from build123d import *

# Parameters (mm, degrees)
F1_DEPTH = 10
F2_DEPTH = 8
F3_DEPTH = 5


with BuildPart() as f1:
    # F0 (on Front) → F1 (new body, symmetric)
    with BuildSketch(Plane.XZ):
        with BuildLine():
            ThreePointArc((3.989783, 27.714286), (0, 24), (-3.989783, 27.714286))
            ThreePointArc((-3.989783, 27.714286), (-9.576564, 26.311393), (-14.758048, 23.794958))
            ThreePointArc((-14.758048, 23.794958), (-15.426903, 18.385067), (-20.87075, 18.665792))
            ThreePointArc((-20.87075, 18.665792), (-24.248711, 14), (-26.600425, 8.741704))
            ThreePointArc((-26.600425, 8.741704), (-23.635386, 4.167556), (-27.986062, 0.883366))
            ThreePointArc((-27.986062, 0.883366), (-27.574617, -4.862149), (-25.996167, -10.40189))
            ThreePointArc((-25.996167, -10.40189), (-20.78461, -12), (-22.006384, -17.312396))
            ThreePointArc((-22.006384, -17.312396), (-17.998053, -21.449244), (-13.228013, -24.678324))
            ThreePointArc((-13.228013, -24.678324), (-8.208483, -22.552623), (-5.729674, -27.407496))
            ThreePointArc((-5.729674, -27.407496), (0, -28), (5.729674, -27.407496))
            ThreePointArc((5.729674, -27.407496), (8.208483, -22.552623), (13.228013, -24.678324))
            ThreePointArc((13.228013, -24.678324), (17.998053, -21.449244), (22.006384, -17.312396))
            ThreePointArc((22.006384, -17.312396), (20.78461, -12), (25.996167, -10.40189))
            ThreePointArc((25.996167, -10.40189), (27.574617, -4.862149), (27.986062, 0.883366))
            ThreePointArc((27.986062, 0.883366), (23.635386, 4.167556), (26.600425, 8.741704))
            ThreePointArc((26.600425, 8.741704), (24.248711, 14), (20.87075, 18.665792))
            ThreePointArc((20.87075, 18.665792), (15.426903, 18.385067), (14.758048, 23.794958))
            ThreePointArc((14.758048, 23.794958), (9.576564, 26.311393), (3.989783, 27.714286))
        make_face()
        with BuildLine():
            ThreePointArc((2, 19.899749), (0, -20), (-2, 19.899749))
            Line((-2, 19.899749), (-2, 21.899749))
            Line((-2, 21.899749), (2, 21.899749))
            Line((2, 21.899749), (2, 19.899749))
        make_face(mode=Mode.SUBTRACT)
    extrude(amount=F1_DEPTH, both=True)



with BuildPart() as f2:
    # F0 (on Front) → F2 (new body, symmetric)
    with BuildSketch(Plane.XZ):
        with BuildLine():
            Line((-10.825318, 78.25), (-15.155445, 80.75))
            ThreePointArc((-15.155445, 80.75), (-17.338404, 74.372706), (-16.949042, 67.643398))
            ThreePointArc((-16.949042, 67.643398), (0, 54.5), (16.949042, 67.643398))
            ThreePointArc((16.949042, 67.643398), (17.338404, 74.372706), (15.155445, 80.75))
            Line((15.155445, 80.75), (10.825318, 78.25))
            ThreePointArc((10.825318, 78.25), (0, 59.5), (-10.825318, 78.25))
        make_face()
        with BuildLine():
            ThreePointArc((-50.10638, -48.5), (-47.198385, -27.25), (-67.055422, -19.143398))
            ThreePointArc((-67.055422, -19.143398), (-73.077855, -22.170855), (-77.509274, -27.25))
            Line((-77.509274, -27.25), (-73.179147, -29.75))
            ThreePointArc((-73.179147, -29.75), (-51.528512, -29.75), (-62.353829, -48.5))
            Line((-62.353829, -48.5), (-62.353829, -53.5))
            ThreePointArc((-62.353829, -53.5), (-55.739451, -52.201852), (-50.10638, -48.5))
        make_face()
        with BuildLine():
            ThreePointArc((77.509274, -27.25), (73.077855, -22.170855), (67.055422, -19.143398))
            ThreePointArc((67.055422, -19.143398), (47.198385, -27.25), (50.10638, -48.5))
            ThreePointArc((50.10638, -48.5), (55.739451, -52.201852), (62.353829, -53.5))
            Line((62.353829, -53.5), (62.353829, -48.5))
            ThreePointArc((62.353829, -48.5), (51.528512, -29.75), (73.179147, -29.75))
            Line((73.179147, -29.75), (77.509274, -27.25))
        make_face()
    extrude(amount=F2_DEPTH, both=True)


with BuildPart() as f1_1:
    add(f1.part)

    add(f2.part)  # F3 merges F2
    # F0 (on Front) → F3 (join, symmetric)
    with BuildSketch(Plane.XZ):
        with BuildLine():
            ThreePointArc((16.949042, 67.643398), (0, 54.5), (-16.949042, 67.643398))
            Line((-16.949042, 67.643398), (-67.055422, -19.143398))
            ThreePointArc((-67.055422, -19.143398), (-47.198385, -27.25), (-50.10638, -48.5))
            Line((-50.10638, -48.5), (50.10638, -48.5))
            ThreePointArc((50.10638, -48.5), (47.198385, -27.25), (67.055422, -19.143398))
            Line((67.055422, -19.143398), (16.949042, 67.643398))
        make_face()
        with BuildLine():
            ThreePointArc((-14.758048, 23.794958), (-9.576564, 26.311393), (-3.989783, 27.714286))
            ThreePointArc((-3.989783, 27.714286), (0, 24), (3.989783, 27.714286))
            ThreePointArc((3.989783, 27.714286), (9.576564, 26.311393), (14.758048, 23.794958))
            ThreePointArc((14.758048, 23.794958), (15.426903, 18.385067), (20.87075, 18.665792))
            ThreePointArc((20.87075, 18.665792), (24.248711, 14), (26.600425, 8.741704))
            ThreePointArc((26.600425, 8.741704), (23.635386, 4.167556), (27.986062, 0.883366))
            ThreePointArc((27.986062, 0.883366), (27.574617, -4.862149), (25.996167, -10.40189))
            ThreePointArc((25.996167, -10.40189), (20.78461, -12), (22.006384, -17.312396))
            ThreePointArc((22.006384, -17.312396), (17.998053, -21.449244), (13.228013, -24.678324))
            ThreePointArc((13.228013, -24.678324), (8.208483, -22.552623), (5.729674, -27.407496))
            ThreePointArc((5.729674, -27.407496), (0, -28), (-5.729674, -27.407496))
            ThreePointArc((-5.729674, -27.407496), (-8.208483, -22.552623), (-13.228013, -24.678324))
            ThreePointArc((-13.228013, -24.678324), (-17.998053, -21.449244), (-22.006384, -17.312396))
            ThreePointArc((-22.006384, -17.312396), (-20.78461, -12), (-25.996167, -10.40189))
            ThreePointArc((-25.996167, -10.40189), (-27.574617, -4.862149), (-27.986062, 0.883366))
            ThreePointArc((-27.986062, 0.883366), (-23.635386, 4.167556), (-26.600425, 8.741704))
            ThreePointArc((-26.600425, 8.741704), (-24.248711, 14), (-20.87075, 18.665792))
            ThreePointArc((-20.87075, 18.665792), (-15.426903, 18.385067), (-14.758048, 23.794958))
        make_face(mode=Mode.SUBTRACT)
    extrude(amount=F3_DEPTH, both=True)


solid = f1_1.part
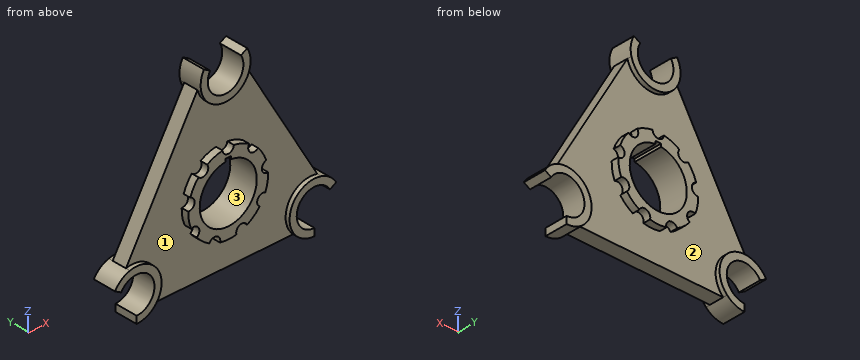
Work out the finished part from the listing and answer in its coordinate system (mm). Face numbers are marked on the shaded views. A direction names the side the tool comes from. Give positions to 0.01 mm unless a question says otherwise; leave off trailing zeros. Loops run counter-clockwise (first coordinate to the right, second up) from the corner with the lowest first, then second, coordinate; pieces in that order, holes last. Notation, with made-up numbers: (51.5, -38) -> (91.5, -38) arc R19 cw to (91.5, -9) -> close; hole circle Ø3 at (51.5, -37.5). An arc over 180 degrees is marked (long way). Use a Markdown table: item, result. Add a question column.
1. Section D-D on z = -36 is taken. Determine the outline of the cut face in (x, y), and give its area (3 significant figures).
2. Section C-C on x = 0 is taken. Determine the outline of the cut face in (y, z).
3. Flat-ended cylindrical pins translate along their axes: pin 1 Ø4 at (y, z) = (0, -50) entering from -X; pin 2 Ø6 at (x, y) = (22, -6) entering from +Z; pin 3 Ø5.5 at (y, z) = (1, -51.5) entering from +X; pin 4 Ø13 at (x, z) = (1.5, 72.5) entering from -Y. Find the tip coordinate at first contact, or state that the pin passes through.
4. Find the intervals of material crossed by probe 1 along X at (y, z) = (-7.5, -22); probe 2 along X at (y, z) = (-1.5, 72); probe 3 along X at (y, z) = (-1.75, -36), in increasing order.
5. For the marked faces 1, 2 and 3, determine the directions among +Z, -Z, +X, -X, +Y, -Y from which every point of the face is accessible in a straight line to the end or side of a thin tool.
6. Section A-A on y = 0.5 is taken. Determine the outline of the cut face in (x, z), and give its area (3 significant figures).
7. Section B-B on z = 72 is taken. Determine the outline of the cut face in (x, y).
Results below:
| question | item | result |
|---|---|---|
| 1 | outline | (-49.85, -8) -> (-44.85, -8) -> (-44.85, -5) -> (44.85, -5) -> (44.85, -8) -> (49.85, -8) -> (49.85, 8) -> (44.85, 8) -> (44.85, 5) -> (-44.85, 5) -> (-44.85, 8) -> (-49.85, 8) -> close |
| 1 | area | 1,060 mm^2 |
| 2 | outline | (-10, -28) -> (-5, -28) -> (-5, -48.5) -> (5, -48.5) -> (5, -28) -> (10, -28) -> (10, -20) -> (-10, -20) -> close; (-10, 21.9) -> (10, 21.9) -> (10, 24) -> (5, 24) -> (5, 54.5) -> (8, 54.5) -> (8, 59.5) -> (-8, 59.5) -> (-8, 54.5) -> (-5, 54.5) -> (-5, 24) -> (-10, 24) -> close |
| 3 | pin 1 | stops at x = -62.35 |
| 3 | pin 2 | stops at z = 63.79 |
| 3 | pin 3 | stops at x = 62.35 |
| 3 | pin 4 | passes through |
| 4 | probe 1 | x = -72.85 to -51.85, -17.32 to 17.32, 51.85 to 72.85 |
| 4 | probe 2 | x = -17.5 to -12.5, 12.5 to 17.5 |
| 4 | probe 3 | x = -49.85 to 49.85 |
| 5 | face 1 | -Y |
| 5 | face 2 | +Y |
| 5 | face 3 | +Y, -Y |
| 6 | outline | (-77.51, -27.25) -> (-73.18, -29.75) arc R12.5 cw (long way) to (-62.35, -48.5) -> (-62.35, -53.5) arc R17.5 ccw to (-50.11, -48.5) -> (50.11, -48.5) arc R17.5 ccw to (62.35, -53.5) -> (62.35, -48.5) arc R12.5 cw (long way) to (73.18, -29.75) -> (77.51, -27.25) arc R17.5 ccw to (67.06, -19.14) -> (16.95, 67.64) arc R17.5 ccw to (15.16, 80.75) -> (10.83, 78.25) arc R12.5 cw (long way) to (-10.83, 78.25) -> (-15.16, 80.75) arc R17.5 ccw to (-16.95, 67.64) -> (-67.06, -19.14) arc R17.5 ccw to start; hole (-2, 19.9) arc R20 ccw (long way) to (2, 19.9) -> (2, 21.9) -> (-2, 21.9) -> close |
| 6 | area | 9,420 mm^2 |
| 7 | outline | (-17.5, -8) -> (-12.5, -8) -> (-12.5, 8) -> (-17.5, 8) -> close; (12.5, -8) -> (17.5, -8) -> (17.5, 8) -> (12.5, 8) -> close |
